Part model, mm, in its own coordinate system. Face numbers are marked on the shaded views. A direction names the side the tool comes from. Coordinates: 2 decimals unless noted, no trailing zeros. Loops run counter-clockwise (first coordinate to the right, second up) from the corner with the lowest first, then second, coordinate; pieces in that order, holes last. Notation, with made-up numbers: (81, 77.5) - (127, 77.5) arc R10 ccw to (127, 81.5) - close; hole circle Ø5 at (0, -30). An arc over 180 degrees is marked (long way). One line per question, with ' | ' between items. Start each with the question number.
from build123d import *

# Parameters (mm, degrees)
SZKIC1_R                    = 4
DODANIE_WYCI_GNI_CIE1_DEPTH = 5.5
SZKIC2_R                    = 6.5
SZKIC2_R_2                  = 4
DODANIE_WYCI_GNI_CIE2_DEPTH = 8
SFAZOWANIE1_SIZE            = 0.75


with BuildPart() as part:
    # Szkic1 → Dodanie-wyciągnięcie1 (new body)
    with BuildSketch(Plane.XY):
        Polygon((-7.505553499, 0), (-3.75277675, -6.5), (3.75277675, -6.5), (7.505553499, 0), (3.75277675, 6.5), (-3.75277675, 6.5), align=None)
        Circle(SZKIC1_R, mode=Mode.SUBTRACT)
    extrude(amount=DODANIE_WYCI_GNI_CIE1_DEPTH)

    # Szkic2 → Dodanie-wyciągnięcie2 (add)
    with BuildSketch(Plane.XY):
        Circle(SZKIC2_R)
        Circle(SZKIC2_R_2, mode=Mode.SUBTRACT)
    extrude(amount=DODANIE_WYCI_GNI_CIE2_DEPTH)

    # Sfazowanie1
    sfazowanie1_edges = [part.edges().sort_by_distance(p)[0] for p in [
        (-4, 0, 0),
        (-4, 0, 8),
    ]]
    chamfer(sfazowanie1_edges, length=SFAZOWANIE1_SIZE)

    # Szkic3 → Wycięcie-obrót1 (revolve, cut)
    with BuildSketch(Plane(origin=(0, 0, 0), x_dir=(1, 0, 0), z_dir=(0, 1, 0))):
        with BuildLine():
            Line((-7.505553499, 0), (-7.505553499, -0.905553499))
            ThreePointArc((-7.505553499, -0.905553499), (-7.24032302, -0.265230479), (-6.6, 0))
            Line((-6.6, 0), (-7.505553499, 0))
        make_face()
        with BuildLine():
            ThreePointArc((-6.6, -5.5), (-7.24032302, -5.234769521), (-7.505553499, -4.594446501))
            Line((-7.505553499, -4.594446501), (-7.505553499, -5.5))
            Line((-7.505553499, -5.5), (-6.6, -5.5))
        make_face()
        with BuildLine():
            Line((-6.5, -8), (-5.25, -8))
            ThreePointArc((-5.25, -8), (-6.133883476, -7.633883476), (-6.5, -6.75))
            Line((-6.5, -6.75), (-6.5, -8))
        make_face()
    revolve(axis=Axis((0, 0, -1.701574894), (0, 0, 1)), mode=Mode.SUBTRACT)


solid = part.part
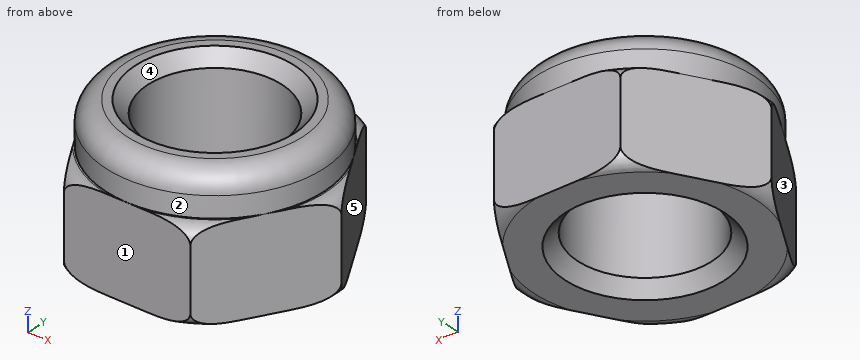
1) Band-saw the part on B-B on z = 5.25. List the corners of the cut face in (x, y).
2) Pin check, flat tips, straight feed: pin 1 Ø1 at (y, z) = (3, 6) entering from +X; pin 2 Ø1.6 at (x, y) = (-4, -5.5) entering from +Z; pin 3 Ø6.5 at (x, y) = (0, 0) entering from -Z; pin 4 Ø0.5 at (x, y) = (-6, -1) entering from +Z. Stop position of each tip, or through.
3) Wall check: line 1 along Y through (x, z) = (0, 5); line 2 along X through (y, z) = (4.25, 4.75); line 3 along X through (y, z) = (-1, 6). Give the ranges that are in metal, low to high. Write a range as [from, to].
4) Mould opens along X. For the marked faces 3, 4 and 5 say: +X half, -X half, draft (parallel to the pull), parting line (faces both ways), or undercut.
5) Band-saw the part on A-A on z = 2. List the corners of the cut face in (x, y).
6) Tool access for the marked faces 1 and 2: list every direction of +Z, -Z, +X, -X, +Y, -Y with a clear straight run to the whole face (end or side of a thin tool).
Values found:
1) outline: (-7.21, -0.52) - (-4.05, -5.98) arc R7.22 ccw to (-3.15, -6.5) - (3.15, -6.5) arc R7.22 ccw to (4.05, -5.98) - (7.21, -0.52) arc R7.22 ccw to (7.21, 0.52) - (4.05, 5.98) arc R7.22 ccw to (3.15, 6.5) - (-3.15, 6.5) arc R7.22 ccw to (-4.05, 5.98) - (-7.21, 0.52) arc R7.22 ccw to start; hole circle Ø8 at (0, 0)
2) pin 1: x = 6 | pin 2: z = 7.75 | pin 3: through | pin 4: z = 7.86
3) line 1: [-6.5, -4], [4, 6.5] | line 2: [-5.05, 5.05] | line 3: [-6.42, -3.87], [3.87, 6.42]
4) face 3: -X half | face 4: undercut | face 5: +X half
5) outline: (-7.51, 0) - (-3.75, -6.5) - (3.75, -6.5) - (7.51, 0) - (3.75, 6.5) - (-3.75, 6.5) - close; hole circle Ø8 at (0, 0)
6) face 1: +Z, -Z, +X, -X, -Y | face 2: +Z
